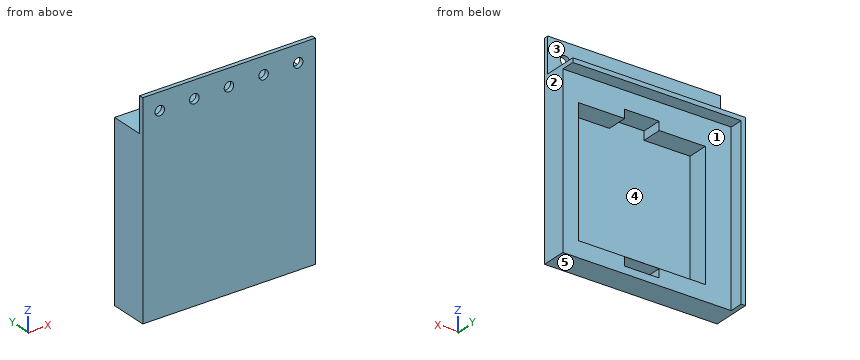
from build123d import *

# Parameters (mm, degrees)
SKETCH1_W               = 304.8
SKETCH1_H               = 304.8
SKETCH1_W_2             = 93
SKETCH1_H_2             = 93
BOSS_EXTRUDE1_DEPTH     = 15.24
SKETCH2_W               = 304.8
SKETCH2_H               = 304.8
BOSS_EXTRUDE2_DEPTH     = 3.175
SKETCH3_W               = 304.8
SKETCH3_H               = 304.8
SKETCH3_W_2             = 247.214
SKETCH3_H_2             = 247.214
BOSS_EXTRUDE3_DEPTH     = 10
SKETCH4_OUTSIDE_W       = 393.198
SKETCH4_OUTSIDE_H       = 393.198
SKETCH4_OUTSIDE_W_2     = 253.564
SKETCH4_OUTSIDE_H_2     = 253.564
CUT_EXTRUDE1_DEPTH      = 25.24
SKETCH5_R               = 3.4925
CUT_EXTRUDE2_DEPTH      = 217.999026726
SKETCH6_W               = 25.4
SKETCH6_H               = 6.35
CUT_EXTRUDE3_DEPTH      = 15.24
LPATTERN1_COUNT         = 2
LPATTERN1_PITCH         = 116.078
LPATTERN1_COUNT_DIR2    = 2
LPATTERN1_PITCH_DIR2    = 116.078
SKETCH7_W               = 388.208697242
SKETCH7_H               = 185.968986832
CUT_EXTRUDE4_DEPTH      = 320.069595424
SKETCH8_W               = 545.051384684
SKETCH8_H               = 463.265958
CUT_EXTRUDE5_DEPTH      = 320.069595424
SKETCH9_W               = 585.539242267
SKETCH9_H               = 383.639310532
CUT_EXTRUDE6_DEPTH      = 297.913320173
CUT_EXTRUDE7_DEPTH      = 200.841169742
CUT_EXTRUDE7_DEPTH_BACK = 200.841169742
SKETCH10_OUTSIDE_W      = 331.206
SKETCH10_OUTSIDE_H      = 356.824
SKETCH10_OUTSIDE_W_2    = 142.114384532
SKETCH10_OUTSIDE_H_2    = 171.89804786


with BuildPart() as part:
    # Sketch1 → Boss-Extrude1 (new body)
    with BuildSketch(Plane(origin=(0, 0, 0), x_dir=(1, 0, 0), z_dir=(0, 1, 0))):
        Rectangle(SKETCH1_W, SKETCH1_H)
        with Locations((58.057, 58.057)):
            Rectangle(SKETCH1_W_2, SKETCH1_H_2, mode=Mode.SUBTRACT)
        with Locations((-58.057, 58.057)):
            Rectangle(SKETCH1_W_2, SKETCH1_H_2, mode=Mode.SUBTRACT)
        with Locations((-58.057, -58.057)):
            Rectangle(SKETCH1_W_2, SKETCH1_H_2, mode=Mode.SUBTRACT)
        with Locations((58.057, -58.057)):
            Rectangle(SKETCH1_W_2, SKETCH1_H_2, mode=Mode.SUBTRACT)
    extrude(amount=BOSS_EXTRUDE1_DEPTH)

    # Sketch2 → Boss-Extrude2 (add)
    with BuildSketch(Plane(origin=(0, 0, 0), x_dir=(-1, 0, 0), z_dir=(0, -1, 0))):
        Rectangle(SKETCH2_W, SKETCH2_H)
    extrude(amount=BOSS_EXTRUDE2_DEPTH)

    # Sketch3 → Boss-Extrude3 (add)
    with BuildSketch(Plane(origin=(0, 15.24, 0), x_dir=(1, 0, 0), z_dir=(0, 1, 0))):
        Rectangle(SKETCH3_W, SKETCH3_H)
        Rectangle(SKETCH3_W_2, SKETCH3_H_2, mode=Mode.SUBTRACT)
    extrude(amount=BOSS_EXTRUDE3_DEPTH)

    # Sketch4 outside → Cut-Extrude1 (cut)
    with BuildSketch(Plane(origin=(0, 25.24, 0), x_dir=(1, 0, 0), z_dir=(0, 1, 0))):
        Rectangle(SKETCH4_OUTSIDE_W, SKETCH4_OUTSIDE_H)
        Rectangle(SKETCH4_OUTSIDE_W_2, SKETCH4_OUTSIDE_H_2, mode=Mode.SUBTRACT)
    extrude(amount=-CUT_EXTRUDE1_DEPTH, mode=Mode.SUBTRACT)

    # Sketch5 → Cut-Extrude2 (cut, through all)
    with BuildSketch(Plane(origin=(0, 0, 0), x_dir=(1, 0, 0), z_dir=(0, 1, 0))):
        with Locations(Location((-139.7, -139.7, 0), (0, 0, 270))):
            Circle(SKETCH5_R)
        with Locations(Location((-114.3, -139.7, 0), (0, 0, 270))):
            Circle(SKETCH5_R)
        with Locations(Location((-88.9, -139.7, 0), (0, 0, 270))):
            Circle(SKETCH5_R)
        with Locations(Location((-63.5, -139.7, 0), (0, 0, 270))):
            Circle(SKETCH5_R)
        with Locations(Location((-38.1, -139.7, 0), (0, 0, 270))):
            Circle(SKETCH5_R)
        with Locations(Location((-12.7, -139.7, 0), (0, 0, 270))):
            Circle(SKETCH5_R)
        with Locations(Location((12.7, -139.7, 0), (0, 0, 270))):
            Circle(SKETCH5_R)
        with Locations(Location((38.1, -139.7, 0), (0, 0, 270))):
            Circle(SKETCH5_R)
        with Locations(Location((63.5, -139.7, 0), (0, 0, 270))):
            Circle(SKETCH5_R)
        with Locations(Location((88.9, -139.7, 0), (0, 0, 270))):
            Circle(SKETCH5_R)
        with Locations(Location((114.3, -139.7, 0), (0, 0, 270))):
            Circle(SKETCH5_R)
        with Locations(Location((139.7, -139.7, 0), (0, 0, 270))):
            Circle(SKETCH5_R)
        with Locations(Location((-139.7, -114.3, 0), (0, 0, 270))):
            Circle(SKETCH5_R)
        with Locations(Location((-139.7, -88.9, 0), (0, 0, 270))):
            Circle(SKETCH5_R)
        with Locations(Location((-139.7, -63.5, 0), (0, 0, 270))):
            Circle(SKETCH5_R)
        with Locations(Location((-139.7, -38.1, 0), (0, 0, 270))):
            Circle(SKETCH5_R)
        with Locations(Location((-139.7, -12.7, 0), (0, 0, 270))):
            Circle(SKETCH5_R)
        with Locations(Location((-139.7, 12.7, 0), (0, 0, 270))):
            Circle(SKETCH5_R)
        with Locations(Location((-139.7, 38.1, 0), (0, 0, 270))):
            Circle(SKETCH5_R)
        with Locations(Location((-139.7, 63.5, 0), (0, 0, 270))):
            Circle(SKETCH5_R)
        with Locations(Location((-139.7, 88.9, 0), (0, 0, 270))):
            Circle(SKETCH5_R)
        with Locations(Location((-139.7, 114.3, 0), (0, 0, 270))):
            Circle(SKETCH5_R)
        with Locations(Location((-139.7, 139.7, 0), (0, 0, 270))):
            Circle(SKETCH5_R)
        with Locations(Location((-114.3, 139.7, 0), (0, 0, 270))):
            Circle(SKETCH5_R)
        with Locations(Location((-88.9, 139.7, 0), (0, 0, 270))):
            Circle(SKETCH5_R)
        with Locations(Location((-63.5, 139.7, 0), (0, 0, 270))):
            Circle(SKETCH5_R)
        with Locations(Location((-38.1, 139.7, 0), (0, 0, 270))):
            Circle(SKETCH5_R)
        with Locations(Location((-12.7, 139.7, 0), (0, 0, 270))):
            Circle(SKETCH5_R)
        with Locations(Location((12.7, 139.7, 0), (0, 0, 270))):
            Circle(SKETCH5_R)
        with Locations(Location((38.1, 139.7, 0), (0, 0, 270))):
            Circle(SKETCH5_R)
        with Locations(Location((63.5, 139.7, 0), (0, 0, 270))):
            Circle(SKETCH5_R)
        with Locations(Location((88.9, 139.7, 0), (0, 0, 270))):
            Circle(SKETCH5_R)
        with Locations(Location((114.3, 139.7, 0), (0, 0, 270))):
            Circle(SKETCH5_R)
        with Locations(Location((139.7, 139.7, 0), (0, 0, 270))):
            Circle(SKETCH5_R)
        with Locations(Location((139.7, 114.3, 0), (0, 0, 270))):
            Circle(SKETCH5_R)
        with Locations(Location((139.7, 88.9, 0), (0, 0, 270))):
            Circle(SKETCH5_R)
        with Locations(Location((139.7, 63.5, 0), (0, 0, 270))):
            Circle(SKETCH5_R)
        with Locations(Location((139.7, 38.1, 0), (0, 0, 270))):
            Circle(SKETCH5_R)
        with Locations(Location((139.7, 12.7, 0), (0, 0, 270))):
            Circle(SKETCH5_R)
        with Locations(Location((139.7, -12.7, 0), (0, 0, 270))):
            Circle(SKETCH5_R)
        with Locations(Location((139.7, -38.1, 0), (0, 0, 270))):
            Circle(SKETCH5_R)
        with Locations(Location((139.7, -63.5, 0), (0, 0, 270))):
            Circle(SKETCH5_R)
        with Locations(Location((139.7, -88.9, 0), (0, 0, 270))):
            Circle(SKETCH5_R)
        with Locations(Location((139.7, -114.3, 0), (0, 0, 270))):
            Circle(SKETCH5_R)
    extrude(amount=-CUT_EXTRUDE2_DEPTH, mode=Mode.SUBTRACT)

    # Sketch6 → Cut-Extrude3 (cut)
    with BuildSketch(Plane(origin=(0, 15.24, 0), x_dir=(1, 0, 0), z_dir=(0, 1, 0))):
        with Locations((-58.057, 107.732)):
            Rectangle(SKETCH6_W, SKETCH6_H)
        with Locations((-58.057, 8.382)):
            Rectangle(SKETCH6_W, SKETCH6_H)
    cut_extrude3 = extrude(amount=-CUT_EXTRUDE3_DEPTH, mode=Mode.SUBTRACT)

    # LPattern1: Cut-Extrude3 2 × 2
    with Locations(*[(i * LPATTERN1_PITCH, 0, j * LPATTERN1_PITCH_DIR2) for i in range(LPATTERN1_COUNT) for j in range(LPATTERN1_COUNT_DIR2) if (i, j) != (0, 0)]):
        add(cut_extrude3, mode=Mode.SUBTRACT)

    # Sketch7 → Cut-Extrude4 (cut, through all)
    with BuildSketch(Plane(origin=(0, 0, -126.782), x_dir=(-1, 0, 0), z_dir=(0, 0, -1))):
        with Locations((-26.237813245, -25.540582214)):
            Rectangle(SKETCH7_W, SKETCH7_H)
    extrude(amount=CUT_EXTRUDE4_DEPTH, mode=Mode.SUBTRACT)

    # Sketch8 → Cut-Extrude5 (cut, through all)
    with BuildSketch(Plane.ZY.offset(126.782)):
        with Locations((35.238029092, 25.908608745)):
            Rectangle(SKETCH8_W, SKETCH8_H)
    extrude(amount=CUT_EXTRUDE5_DEPTH, mode=Mode.SUBTRACT)

    # Sketch9 → Cut-Extrude6 (cut, through all)
    with BuildSketch(Plane(origin=(126.782, 0, 0), x_dir=(0, 0, -1), z_dir=(1, 0, 0))):
        with Locations((26.844145207, 44.758305083)):
            Rectangle(SKETCH9_W, SKETCH9_H)
    extrude(amount=CUT_EXTRUDE6_DEPTH, mode=Mode.SUBTRACT)

    # Sketch10 outside → Cut-Extrude7 (cut, two sides: drawn at the far end of the back side and taken through both)
    with BuildSketch(Plane(origin=(0, 0, 0), x_dir=(1, 0, 0), z_dir=(0, 1, 0)).offset(-CUT_EXTRUDE7_DEPTH_BACK)):
        with Locations((0, -12.809)):
            Rectangle(SKETCH10_OUTSIDE_W, SKETCH10_OUTSIDE_H)
        with Locations((-71.057192266, -85.94902393)):
            Rectangle(SKETCH10_OUTSIDE_W_2, SKETCH10_OUTSIDE_H_2, mode=Mode.SUBTRACT)
    extrude(amount=CUT_EXTRUDE7_DEPTH + CUT_EXTRUDE7_DEPTH_BACK, mode=Mode.SUBTRACT)


solid = part.part
For this review, take the finished solid that the model builds, in its own axes (mm). Face numbers are marked on the shaded views. A direction names the side the tool comes from. Give positions to 0.01 mm unless a question says otherwise; leave off trailing zeros. Loops run counter-clockwise (first coordinate to the right, second up) from the corner with the lowest first, then second, coordinate; pieces in that order, holes last.
Item 1: Take a section at A-A, the plane x = -38.1. State the section outline as (y, z) points (1 decimal).
Item 2: Take a section at C-C, the plane y = 4.5. State the section outline as (x, z) points, and give its area (3 significant figures).
Item 3: Draft analysis for pull direction Z (two halves, no side actions). For the marked faces 3, 4 and 5, state which applies: +Z half, -Z half, draft (parallel to the pull), parting line (faces both ways), or undercut.
Item 4: Insertion check: pin 1 (3 mm diameter, centred on x = -69, y = 19, fed in from -Z); pin 2 (1.5 mm diameter, centred on x = -107.5, z = 114, fed in from +Y); pin 3 (7.5 mm diameter, centred on x = -63, y = 7, fed in from +Z). Each pin has a flat end and moves straight along its axis. Give the tip position at first contact, or say it passes through.
Item 5: Take a section at B-B, the plane z = 139.7. State the section outline as (x, y) points (1 decimal), and give its area (3 significant figures).
Item 6: For line 1 along X through (y, z) = (-1.6, 139.7); line 2 along Z through (x, y) = (-95, 11.75); line 3 along X through (y, z) = (5.25, 57), list the stretches that pass through material, from the lowest coordinate up.
Item 7: Take a section at D-D, the plane x = -52.5. State the section outline as (y, z) points (3 decimals).
Item 8: Tool access review of the marked faces 1 and 2: name each direction out of +Z, -Z, +X, -X, +Y, -Y from which nothing blocks a thin tool from reaching the whole face with its end or side.
Calculated:
1. outline: (-3.2, 0) - (15.2, 0) - (15.2, 11.6) - (0, 11.6) - (0, 104.6) - (15.2, 104.6) - (15.2, 123.6) - (25.2, 123.6) - (25.2, 126.8) - (0, 126.8) - (0, 136.2) - (-3.2, 136.2) - close; (-3.2, 143.2) - (0, 143.2) - (0, 152.4) - (-3.2, 152.4) - close
2. outline: (-126.78, 0) - (0, 0) - (0, 126.78) - (-126.78, 126.78) - close; hole (-104.56, 11.56) - (-11.56, 11.56) - (-11.56, 104.56) - (-45.36, 104.56) - (-45.36, 110.87) - (-70.76, 110.87) - (-70.76, 104.56) - (-104.56, 104.56) - close; hole (-70.76, 5.17) - (-45.36, 5.17) - (-45.36, 11.52) - (-70.76, 11.52) - close
2. area: 7,100 mm2
3. face 3: draft
3. face 4: undercut
3. face 5: -Z half
4. pin 1: stops at z = 123.61
4. pin 2: stops at y = 15.24
4. pin 3: stops at z = 126.78
5. outline: (-126.8, -3.2) - (-117.8, -3.2) - (-117.8, 0) - (-126.8, 0) - close; (-110.8, -3.2) - (-92.4, -3.2) - (-92.4, 0) - (-110.8, 0) - close; (-85.4, -3.2) - (-67, -3.2) - (-67, 0) - (-85.4, 0) - close; (-60, -3.2) - (-41.6, -3.2) - (-41.6, 0) - (-60, 0) - close; (-34.6, -3.2) - (-16.2, -3.2) - (-16.2, 0) - (-34.6, 0) - close; (-9.2, -3.2) - (0, -3.2) - (0, 0) - (-9.2, 0) - close
5. area: 292 mm2
6. line 1: x = -126.78 to -117.79, -110.81 to -92.39, -85.41 to -66.99, -60.01 to -41.59, -34.61 to -16.19, -9.21 to 0
6. line 2: z = 0 to 11.56, 104.56 to 126.78
6. line 3: x = -126.78 to -104.56, -11.56 to 0
7. outline: (-3.175, 0) - (15.24, 0) - (15.24, 5.171) - (0, 5.171) - (0, 11.521) - (15.24, 11.521) - (15.24, 11.557) - (0, 11.557) - (0, 110.871) - (15.24, 110.871) - (15.24, 123.607) - (25.24, 123.607) - (25.24, 126.782) - (0, 126.782) - (0, 152.4) - (-3.175, 152.4) - close
8. face 1: -Z, +X, +Y
8. face 2: +Z, -Z, +X, +Y, -Y
